Could you check a few things on this drawing? It's one solid part, dimensions in mm from its lowest x, y, z. A direction names the side the tool comes from. Give positions to 0.01 mm unless a question says otherwise; leave off trailing zeros. Order: outer loops, then holes, each group sorted by start corner. A loop starts at its lowest first (then second) coordinate and runs counter-clockwise, first axis right, second up. Notation, with made-up numbers: (4.5, 32.25) - (22.5, 32.25) arc R30 ccw to (22.5, 54.25) - close; hole circle Ø2 at (-5.75, 69.5). An arc over 180 degrees is marked (long way). Put each result on its own line as item: value.
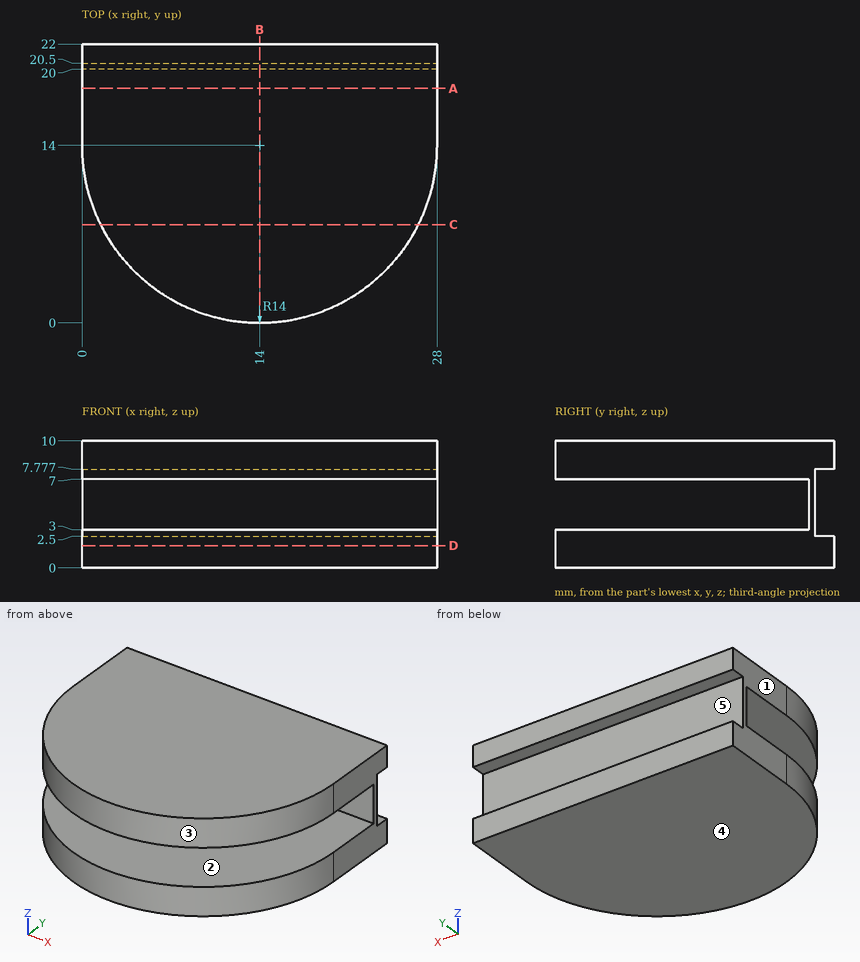
1) Which directions (+Z, -Z, +X, -X, +Y, -Y) give clear straight access to the entire face, cutting with the end or side of a thin tool? Please do the marked faces 1 and 2.
Filled in:
face 1: +Z, -Z, -X, +Y, -Y
face 2: +X, -X, -Y
2) Suppose I cut it at C-C, the plane y = 7.75. List the corners of the cut face in (x, z) for me.
Filled in:
outline: (1.47, 0) - (26.53, 0) - (26.53, 3) - (1.47, 3) - close; (1.47, 7) - (26.53, 7) - (26.53, 10) - (1.47, 10) - close
3) If I drill on line 1 (Z direction, x = 10.25, y = 19.5); line 2 (Y direction, x = 3.25, z = 4.5); line 3 (Y direction, x = 7.75, z = 1.5), over which ranges is the centre line in solid material (lowest first)? Write a range as [from, to].
Filled in:
line 1: z = [0, 3], [7, 10]
line 2: y = [20, 20.5]
line 3: y = [1.47, 22]
4) I'm going to push flat-ended pins straight in: pin 1 (4 mm diameter, centred on x = 21, z = 5, fed in from +Y); pin 2 (4.5 mm diameter, centred on x = 10.5, z = 5, fed in from -Y). Where does each tip first touch, or does it pass through?
Filled in:
pin 1: stops at y = 20.5
pin 2: stops at y = 0.22
5) Suppose I cut it at A-A, the plane y = 18.5. List the corners of the cut face in (x, z) for me, and give its area (3 significant figures).
Filled in:
outline: (0, 0) - (28, 0) - (28, 3) - (0, 3) - close; (0, 7) - (28, 7) - (28, 10) - (0, 10) - close
area: 168 mm^2
6) Suppose I cut it at D-D, the plane z = 1.75. List the corners of the cut face in (x, y) for me, and give its area (3 significant figures).
Filled in:
outline: (0, 14) arc R14 ccw to (28, 14) - (28, 22) - (0, 22) - close
area: 532 mm^2
7) Suppose I cut it at B-B, the plane x = 14. List the corners of the cut face in (y, z) for me, and give its area (3 significant figures).
Filled in:
outline: (0, 0) - (22, 0) - (22, 2.5) - (20.5, 2.5) - (20.5, 7.78) - (22, 7.78) - (22, 10) - (0, 10) - (0, 7) - (20, 7) - (20, 3) - (0, 3) - close
area: 132 mm^2
8) We'd pull the mould along Z, two halves only. Please class the marked faces 3, 4 and 5: pulls with the +Z half, pulls with the -Z half, needs draft (parallel to the pull), parting line crosses it, or undercut.
Filled in:
face 3: needs draft
face 4: pulls with the -Z half
face 5: undercut
